The listing builds one solid part. Answer for the finished solid, in the listing's coordinates (mm). A direction names the side the tool comes from. Round coordinates to 2 decimals unless told otherwise and drop trailing zeros. Order: outer loops, then holes, each group sorted by start corner. A loop starts at its lowest first (then second) coordinate and runs counter-clockwise, first axis right, second up. Notation, with made-up numbers: (-8, -6.75) -> (32, -6.75) arc R29 ccw to (32, 19.25) -> close; hole circle Ø8 at (71.5, 68). An arc over 180 degrees is marked (long way). Answer in a Markdown table with one row per item. Add a question column.
```python
from build123d import *

# Parameters (mm, degrees)
SKETCH1_R                = 12.7
BOSS_EXTRUDE1_DEPTH      = 25.4
BOSS_EXTRUDE2_DEPTH      = 25.4
BOSS_EXTRUDE2_DEPTH_BACK = 25.4
SKETCH2_W                = 50.8
SKETCH2_H                = 38.1
SKETCH3_R                = 6.35
CUT_EXTRUDE1_DEPTH       = 154.454683865
SKETCH4_R                = 12.7
CUT_EXTRUDE2_DEPTH       = 12.7
SKETCH5_R                = 12.7
BOSS_EXTRUDE3_DEPTH      = 152.4
SKETCH6_R                = 31.75
BOSS_EXTRUDE4_DEPTH      = 25.4
FILLET1_R                = 12.7


with BuildPart() as part:
    # Sketch1 → Boss-Extrude1 (new body)
    with BuildSketch(Plane.XY):
        with BuildLine():
            Line((-114.3, 25.4), (114.3, 25.4))
            ThreePointArc((114.3, 25.4), (139.7, 0), (114.3, -25.4))
            Line((114.3, -25.4), (-114.3, -25.4))
            ThreePointArc((-114.3, -25.4), (-139.7, 0), (-114.3, 25.4))
        make_face()
        with Locations((-114.3, 0)):
            Circle(SKETCH1_R, mode=Mode.SUBTRACT)
        with Locations((114.3, 0)):
            Circle(SKETCH1_R, mode=Mode.SUBTRACT)
    extrude(amount=BOSS_EXTRUDE1_DEPTH)

    # Sketch2 → Boss-Extrude2 (add, two sides: drawn at the far end of the back side and taken through both)
    with BuildSketch(Plane(origin=(0, 0, 0), x_dir=(1, 0, 0), z_dir=(0, 1, 0)).offset(-BOSS_EXTRUDE2_DEPTH_BACK)):
        with Locations((0, 19.05)):
            Rectangle(SKETCH2_W, SKETCH2_H)
    extrude(amount=BOSS_EXTRUDE2_DEPTH + BOSS_EXTRUDE2_DEPTH_BACK)

    # Sketch3 → Cut-Extrude1 (cut, through all)
    with BuildSketch(Plane(origin=(0, 25.4, 0), x_dir=(1, 0, 0), z_dir=(0, 1, 0))):
        with Locations(Location((0, 0, 0), (0, 0, 270))):
            Circle(SKETCH3_R)
    extrude(amount=-CUT_EXTRUDE1_DEPTH, mode=Mode.SUBTRACT)

    # Sketch4 → Cut-Extrude2 (cut)
    with BuildSketch(Plane(origin=(0, 0, -38.1), x_dir=(-1, 0, 0), z_dir=(0, 0, -1))):
        Circle(SKETCH4_R)
    extrude(amount=-CUT_EXTRUDE2_DEPTH, mode=Mode.SUBTRACT)

    # Sketch5 → Boss-Extrude3 (add)
    with BuildSketch(Plane(origin=(0, 0, -38.1), x_dir=(-1, 0, 0), z_dir=(0, 0, -1))):
        with Locations((114.3, 0)):
            Circle(SKETCH5_R)
        with Locations((-114.3, 0)):
            Circle(SKETCH5_R)
    extrude(amount=-BOSS_EXTRUDE3_DEPTH)

    # Sketch6 → Boss-Extrude4 (add)
    with BuildSketch(Plane.XY.offset(114.3)):
        with Locations((-114.3, 0)):
            Circle(SKETCH6_R)
        with Locations((114.3, 0)):
            Circle(SKETCH6_R)
    extrude(amount=BOSS_EXTRUDE4_DEPTH)

    # Fillet1
    fillet1_edges = [part.edges().sort_by_distance(p)[0] for p in [
        (-146.05, 0, 114.3),
        (82.55, 0, 114.3),
    ]]
    fillet(fillet1_edges, radius=FILLET1_R)


solid = part.part
```
Item 1: The part is cut by section C-C, the plane x = -53. Give the vertices of the cut face in (y, z), and give its area (3 significant figures).
Item 2: The part is cut by section B-B, the plane z = 90. Give the vertices of the cut face in (x, y), and give its area (3 significant figures).
Item 3: Find the intervals of material crossed by probe 1 along Y at (x, z) = (0, -33); probe 2 along X at (y, z) = (4.5, -26); probe 3 along Z at (x, y) = (53, 6.5), in increasing order. Write a range as [from, to].
Item 4: The part is cut by section A-A, the plane x = 0. Give the vertices of the cut face in (y, z).
Item 5: For a pull along Z with two mould halves and no side action, classify faces 4 (the face through (114, 0, 139.7)), 5 (the face through (2, 0, 25.4)), 6 (the face through (124.4, -7.7, -19.3)), 7 (the face through (118.3, -12.4, 114.3)) as released by +Z, released by -Z, zero draft, split by the parting line, or undercut.
Item 6: Flat-ended cylindrical pins translate along their axes: P1, Ø3, axis at x = 98, y = 14.5, coming from the -Z side; P2, Ø3, axis at x = -85.5, y = 22, coming from the +Z side; P3, Ø6, axis at x = -58, z = 17.5, coming from the -Y side. Find the tip coordinate at first contact, or state that the pin passes through.
Item 7: A tool of negligible diameter and unlimited length cuts with its end or side. For faces 1 (the face through (-101.612, 0.558, -19.317)), 2 (the face through (-2, 25.4, 7)), 3 (the face through (-25.4, 0, -19)), from which of +Z, -Z, +X, -X, +Y, -Y can it reach the whole face along a straight path? Write none if from no direction.
Item 8: The part is cut by section D-D, the plane z = 118.5. Give the vertices of the cut face in (x, y), and give its area (3 significant figures).
Resolved:
| question | item | result |
|---|---|---|
| 1 | outline | (-25.4, 0) -> (25.4, 0) -> (25.4, 25.4) -> (-25.4, 25.4) -> close |
| 1 | area | 1,290 mm2 |
| 2 | outline | circle Ø25.4 at (-114.3, 0); circle Ø25.4 at (114.3, 0) |
| 2 | area | 1,010 mm2 |
| 3 | probe 1 | [-25.4, -12.7], [12.7, 25.4] |
| 3 | probe 2 | [-126.18, -102.42], [-25.4, -11.88], [11.88, 25.4], [102.42, 126.18] |
| 3 | probe 3 | [0, 25.4] |
| 4 | outline | (-25.4, -38.1) -> (-12.7, -38.1) -> (-12.7, -25.4) -> (12.7, -25.4) -> (12.7, -38.1) -> (25.4, -38.1) -> (25.4, -6.35) -> (-25.4, -6.35) -> close; (-25.4, 6.35) -> (25.4, 6.35) -> (25.4, 25.4) -> (-25.4, 25.4) -> close |
| 5 | face 4 | released by +Z |
| 5 | face 5 | undercut |
| 5 | face 6 | zero draft |
| 5 | face 7 | undercut |
| 6 | P1 | z = 0 |
| 6 | P2 | z = 25.4 |
| 6 | P3 | y = -25.4 |
| 7 | face 1 | -Z |
| 7 | face 2 | -Z, +X, -X, +Y |
| 7 | face 3 | -Z, +Y, -Y |
| 8 | outline | circle Ø56.97 at (-114.3, 0); circle Ø56.97 at (114.3, 0) |
| 8 | area | 5,100 mm2 |
